from build123d import *

# Parameters (mm, degrees)
F1_DEPTH = 434.848
F2_W     = 11.3987904478
F2_H     = 6.35
F3_DEPTH = 25.4
F4_R     = 1.6383
F5_DEPTH = 25.4
F6_R     = 1.6383
F7_DEPTH = 25.4


with BuildPart() as f1:
    # F0 (on Right) → F1 (new body)
    with BuildSketch(Plane.YZ):
        with BuildLine():
            ThreePointArc((0, -1.778), (-0.5207641431, -0.5207641431), (-1.778, 0))
            Line((-1.778, 0), (-206.756, 0))
            ThreePointArc((-206.756, 0), (-208.0132358569, -0.5207641431), (-208.534, -1.778))
            Line((-208.534, -1.778), (-208.534, -9.144))
            Line((-208.534, -9.144), (-206.502, -9.144))
            Line((-206.502, -9.144), (-206.502, -2.032))
            Line((-206.502, -2.032), (-1.9587501884, -2.032))
            Line((-1.9587501884, -2.032), (-2.032, -131.4196))
            Line((-2.032, -131.4196), (0, -131.4196))
            Line((0, -131.4196), (0, -1.778))
        make_face()
    extrude(amount=F1_DEPTH)

    # F2 (on face) → F3 (cut)
    with BuildSketch(Plane.XZ.offset(208.534)):
        with Locations((18.2723952239, -5.969)):
            Rectangle(F2_W, F2_H)
    extrude(amount=-F3_DEPTH, mode=Mode.SUBTRACT)

    # F4 (on face) → F5 (cut)
    with BuildSketch(Plane(origin=(0, -1.9575991909, 0.0011082497), x_dir=(1, 0, 0), z_dir=(0, -0.9999998398, 0.0005661269))):
        with Locations((5.969, -125.4517293099)):
            Circle(F4_R)
        with Locations((428.625, -125.4517293099)):
            Circle(F4_R)
    extrude(amount=-F5_DEPTH, mode=Mode.SUBTRACT)

    # F6 (on face) → F7 (cut)
    with BuildSketch(Plane(origin=(0, 0, 0), x_dir=(-1, 0, 0), z_dir=(0, 1, 0))):
        with Locations((-428.625, -7.747)):
            Circle(F6_R)
        with Locations((-5.969, -7.747)):
            Circle(F6_R)
    extrude(amount=-F7_DEPTH, mode=Mode.SUBTRACT)


solid = f1.part
Source: CAD feature listing. Evaluate the final solid. Frame: model axes, mm. A direction names the side the tool comes from. Round coordinates to 2 decimals unless told otherwise and drop trailing zeros. Loops run counter-clockwise (first coordinate to the right, second up) from the corner with the lowest first, then second, coordinate; pieces in that order, holes last.
Q1. Ray query, line 1 (Y direction, x = 318, z = -6); line 2 (Z direction, x = 282, y = -153); line 3 (Y direction, x = 94, z = -80.5). Return the intervals inside material, ascending.
Q2. Section A-A, the plane x = 150.5. Return loops of the section in (y, z).
Q3. First-contact query: P1, Ø0.6, axis at x = 5.5, y = -207, coming from the -Z side; P2, Ø4, axis at x = 222.5, z = -41.5, coming from the -Y side; P3, Ø1.6, axis at x = 20.5, y = -207, coming from the -Z side. Flat tips, straight axial feed; report the tip coordinate or a pass-through.
Q4. Access query for faces 1 (the face through (214, -103, 0)), 2 (the face through (214, -106, -2.032)). Directions: +Z, -Z, +X, -X, +Y, -Y. A direction counts if a zero-diameter tool reaches every point of the face in a straight line with its end or side. Return the directions, or none.
Q5. Section B-B, the plane y = -90. Return loops of the section in (x, z), plus the area to 3 significant figures.
Q6. Section C-C, the plane z = -104.5. Return loops of the section in (x, y), plus the area to 3 significant figures.
Solutions:
1. line 1: y = -208.53 to -206.5, -1.96 to 0
1. line 2: z = -2.03 to 0
1. line 3: y = -2 to 0
2. outline: (-208.53, -9.14) - (-206.5, -9.14) - (-206.5, -2.03) - (-1.96, -2.03) - (-2.03, -131.42) - (0, -131.42) - (0, -1.78) arc R1.78 ccw to (-1.78, 0) - (-206.76, 0) arc R1.78 ccw to (-208.53, -1.78) - close
3. P1: stops at z = -9.14
3. P2: stops at y = -1.98
3. P3: stops at z = -2.79
4. face 1: +Z, +X, -X, +Y, -Y
4. face 2: -Z, +X, -X
5. outline: (0, -2.03) - (434.85, -2.03) - (434.85, 0) - (0, 0) - close
5. area: 884 mm2
6. outline: (0, -2.02) - (434.85, -2.02) - (434.85, 0) - (0, 0) - close
6. area: 877 mm2
